Autodesk Inventor part; units mm, degrees
ref_plane "YZ Plane" through (0, 0, 0) normal (1, 0, 0) x (0, 1, 0)
ref_plane "XZ Plane" through (0, 0, 0) normal (0, 1, 0) x (-1, 0, 0)
ref_plane "XY Plane" through (0, 0, 0) normal (0, 0, 1) x (1, 0, 0)
sketch "Sketch1" plane through (0, 0, 0) normal (0, 1, 0) x (-1, 0, 0)
  line L0 (-7.5, 7.5) -> (7.5, 7.5)
  line L1 (7.5, 7.5) -> (7.5, -7.5)
  line L2 (7.5, -7.5) -> (-7.5, -7.5)
  line L3 (-7.5, -7.5) -> (-7.5, 7.5)
  line L4 (-7.5, 7.5) -> (7.5, -7.5) construction
  line L5 (7.5, 7.5) -> (-7.5, -7.5) construction
  point P0 (0, 0)
  dimension "d0" = 15
  dimension "d1" = 15
extrude "Extrusion1" add sketch "Sketch1" along normal blind 4
sketch "Sketch2" plane through (0, 4, 0) normal (0, 1, 0) x (1, 0, 0)
  line L0 (5.5, -5.5) -> (-5.5, -5.5) construction
  line L1 (-5.5, -5.5) -> (-5.5, 5.5) construction
  line L2 (-5.5, 5.5) -> (5.5, 5.5) construction
  line L3 (5.5, 5.5) -> (5.5, -5.5) construction
  line L4 (5.5, -5.5) -> (-5.5, 5.5) construction
  line L5 (-5.5, -5.5) -> (5.5, 5.5) construction
  point P0 (0, 0)
  dimension "d4" = 11
  dimension "d5" = 11
chamfer "Chamfer1" distance 1 angle 45 4 edges at (-7.5, 2, 7.5) (7.5, 2, 7.5) (7.5, 2, -7.5) (-7.5, 2, -7.5)
hole "Hole1" at (-5.5, 4, -5.5) at (5.5, 4, -5.5) at (5.5, 4, 5.5) at (-5.5, 4, 5.5) direction (0, -1, 0) diameter 1.6 end through all counterbore diameter 3.1 counterbore depth 1.6
sketch "Sketch3" plane through (0, 4, 0) normal (0, 1, 0) x (1, 0, 0)
  circle A0 centre (0, 0) radius 6
  circle A1 centre (0, 0) radius 4.5
  dimension "d16" = 12
  dimension "d17" = 9
extrude "Extrusion2" cut sketch "Sketch3" against normal blind 0.2
sketch "Sketch4" plane through (0, 0, 0) normal (0, -1, 0) x (1, 0, 0)
  line L0 (-6.5, 7.5) -> (6.5, 7.5)
  line L1 (-3, -7.5) -> (3, -7.5)
  line L2 (3, -7.5) -> (3, 7.5)
  line L3 (3, 7.5) -> (-3, 7.5)
  line L4 (-3, 7.5) -> (-3, -7.5)
  line L5 (-3, -7.5) -> (3, 7.5) construction
  line L6 (3, -7.5) -> (-3, 7.5) construction
  line L7 (7.5, 6.5) -> (7.5, -6.5)
  line L8 (-7.5, -3) -> (7.5, -3)
  line L9 (7.5, -3) -> (7.5, 3)
  line L10 (7.5, 3) -> (-7.5, 3)
  line L11 (-7.5, 3) -> (-7.5, -3)
  line L12 (-7.5, -3) -> (7.5, 3) construction
  line L13 (7.5, -3) -> (-7.5, 3) construction
  point P0 (0, 0)
  point P1 (-3, -3)
  point P2 (3, -3)
  point P3 (3, 3)
  point P4 (-3, 3)
  dimension "d20" = 6
  dimension "d21" = 6
extrude "Extrusion3" cut sketch "Sketch4" against normal blind 0.3
properties part number "D-100.00 Capacitive Sensor" material "Aluminum 6061"
Here's how the part is built. I have some questions about the finished solid (model axes, mm). A direction names the side the tool comes from. Give positions to 0.01 mm unless a question says otherwise; leave off trailing zeros. Loops run counter-clockwise (first coordinate to the right, second up) from the corner with the lowest first, then second, coordinate; pieces in that order, holes last. Notation, with made-up numbers: M -26.75,-2.75 L -8.75,-2.75 A21 cw -8.75,18.25 Z; hole C -36,89.5 d7. An arc over 180 degrees is marked long. Use one line per item in the form item = value. Start each with the question number.
Q1. Which directions (+Z, -Z, +X, -X, +Y, -Y) give clear straight access to the entire face, cutting with the end or side of a thin tool? Please do faces 1 (the flat face through (6.2, 2.4, 6.2)), 2 (the flat face through (7, 2, 7)).
Q2. I need wall thicknesses on line 1 along Z through (x, y) = (-5.5, 2.8); line 2 along Z through (x, y) = (0, 3.9); line 3 along X through (y, z) = (0.7, -5.5). Which ranges of each line are inside material? Lowest first, please.
Q3. If we section it at B-B (z = 0): Write out the boundary of the cut face in (x, y).
Q4. Thinking about a two-plate mould opening in Z: for faces 3 (the flat face through (4.8, 0, 4.8)), 4 (the cylindrical face through (5.43, 3.19, 3.95)), 5 (the flat face through (-7, 2, 7)), which applies, +Z half, -Z half, draft (parallel to the pull), parting line (faces both ways), or undercut?
Q5. If we section it at A-A (x = 5.5): Write out the boundary of the cut face in (y, z).
Q6. If we section it at D-D (z = 5.25): Write out the boundary of the cut face in (x, y).
Q7. If we section it at C-C (y = 0.7): Write out the boundary of the cut face in (x, z).
Q8. Will this pin go through, and if not, where does the flat tip stop? pin 1 Ø2.5 at (x, z) = (-5.5, 5.5) entering from +Y.
Taken from the geometry:
q1.face_1 = +Y
q1.face_2 = +Z, +X, +Y, -Y
q2.line_1 = -7.5 to -7.05, -3.95 to 3.95, 7.05 to 7.5
q2.line_2 = -7.5 to -6, -4.5 to 4.5, 6 to 7.5
q2.line_3 = -7.5 to -6.3, -4.7 to 4.7, 6.3 to 7.5
q3.outline = M -7.5,0.3 L 7.5,0.3 L 7.5,4 L 6,4 L 6,3.8 L 4.5,3.8 L 4.5,4 L -4.5,4 L -4.5,3.8 L -6,3.8 L -6,4 L -7.5,4 Z
q4.face_3 = draft
q4.face_4 = undercut
q4.face_5 = +Z half
q5.outline = M 0,-7.5 L 4,-7.5 L 4,-7.05 L 2.4,-7.05 L 2.4,-6.3 L 0,-6.3 Z; M 0,-4.7 L 2.4,-4.7 L 2.4,-3.95 L 4,-3.95 L 4,-2.4 L 3.8,-2.4 L 3.8,2.4 L 4,2.4 L 4,3.95 L 2.4,3.95 L 2.4,4.7 L 0,4.7 L 0,3 L 0.3,3 L 0.3,-3 L 0,-3 Z; M 0,6.3 L 2.4,6.3 L 2.4,7.05 L 4,7.05 L 4,7.5 L 0,7.5 Z
q6.outline = M -7.5,0 L -6.26,0 L -6.26,2.4 L -7.03,2.4 L -7.03,4 L -7.5,4 Z; M -4.74,0 L -3,0 L -3,0.3 L 3,0.3 L 3,0 L 4.74,0 L 4.74,2.4 L 3.97,2.4 L 3.97,4 L 2.9,4 L 2.9,3.8 L -2.9,3.8 L -2.9,4 L -3.97,4 L -3.97,2.4 L -4.74,2.4 Z; M 6.26,0 L 7.5,0 L 7.5,4 L 7.03,4 L 7.03,2.4 L 6.26,2.4 Z
q7.outline = M -7.5,-6.5 L -6.5,-7.5 L 6.5,-7.5 L 7.5,-6.5 L 7.5,6.5 L 6.5,7.5 L -6.5,7.5 L -7.5,6.5 Z; hole C -5.5,-5.5 d1.6; hole C -5.5,5.5 d1.6; hole C 5.5,-5.5 d1.6; hole C 5.5,5.5 d1.6
q8.pin_1 = 2.4
